from build123d import *

# Parameters (mm, degrees)
SKETCH2_W           = 76
SKETCH2_H           = 178
BOSS_EXTRUDE1_DEPTH = 0.9
SKETCH4_R           = 2.667
CUT_EXTRUDE1_DEPTH  = 2
SKETCH5_R           = 2.667
SKETCH5_R_2         = 1.5
BOSS_EXTRUDE2_DEPTH = 0.254
CHAMFER1_SIZE       = 3


with BuildPart() as part:
    # Sketch2 → Boss-Extrude1 (new body)
    with BuildSketch(Plane.XY):
        with Locations((38, 89)):
            Rectangle(SKETCH2_W, SKETCH2_H)
    extrude(amount=BOSS_EXTRUDE1_DEPTH)

    # Sketch4 → Cut-Extrude1 (cut)
    with BuildSketch(Plane.XY.offset(0.9)):
        with Locations((4, 173)):
            Circle(SKETCH4_R)
        with Locations((72, 173)):
            Circle(SKETCH4_R)
        with Locations((72, 5)):
            Circle(SKETCH4_R)
        with Locations((4, 5)):
            Circle(SKETCH4_R)
    extrude(amount=-CUT_EXTRUDE1_DEPTH, mode=Mode.SUBTRACT)

    # Sketch5 → Boss-Extrude2 (add)
    # profile 1 of 4: a face of its own
    with BuildSketch(Plane.XY.offset(0.9)):
        with Locations((4, 5)):
            Circle(SKETCH5_R)
        with Locations(Location((4, 5, 0), (0, 0, 180))):
            Circle(SKETCH5_R_2, mode=Mode.SUBTRACT)
    # profile 2 of 4: a face of its own
    with BuildSketch(Plane.XY.offset(0.9)):
        with Locations((4, 173)):
            Circle(SKETCH5_R)
        with Locations((4, 173)):
            Circle(SKETCH5_R_2, mode=Mode.SUBTRACT)
    # profile 3 of 4: a face of its own
    with BuildSketch(Plane.XY.offset(0.9)):
        with Locations((72, 5)):
            Circle(SKETCH5_R)
        with Locations((72, 5)):
            Circle(SKETCH5_R_2, mode=Mode.SUBTRACT)
    # profile 4 of 4: a face of its own
    with BuildSketch(Plane.XY.offset(0.9)):
        with Locations((72, 173)):
            Circle(SKETCH5_R)
        with Locations(Location((72, 173, 0), (0, 0, 180))):
            Circle(SKETCH5_R_2, mode=Mode.SUBTRACT)
    extrude(amount=-BOSS_EXTRUDE2_DEPTH)

    # Chamfer1
    chamfer1_edges = [part.edges().sort_by_distance(p)[0] for p in [
        (0, 178, 0.45),
        (76, 178, 0.45),
        (76, 0, 0.45),
        (0, 0, 0.45),
    ]]
    chamfer(chamfer1_edges, length=CHAMFER1_SIZE)


solid = part.part
Verification items for the finished model (mm, model axes). A direction names the side the tool comes from. Round coordinates to 2 decimals unless told otherwise and drop trailing zeros.
1. Release check for a two-part mould opening along Y. For faces 1 (the flat face through (37, 90, 0)), 2 (the cylindrical face through (73.43, 175.25, 0.33)), 3 (the flat face through (1.5, 1.5, 0.4)) record: +Y half, -Y half, draft (parallel to the pull), parting line (faces both ways), or undercut.
Final values:
face 1: draft
face 2: undercut
face 3: -Y half
2. Thickness scan on L1, parallel to X at y = 173, z = 0.35; L2, parallel to Y at x = 72, z = 0.8; L3, parallel to Y at x = 72, z = 0.45. Record the ranges inside material, lowest first.
Final values:
L1: x = 0 to 1.33, 6.67 to 69.33, 74.67 to 76
L2: y = 0 to 3.5, 6.5 to 171.5, 174.5 to 178
L3: y = 0 to 2.33, 7.67 to 170.33, 175.67 to 178
3. Go/stop test with a flat-tipped pin: P1, Ø2.5, axis at x = 4.5, y = 5, coming from the -Z side. Record where the tip stops, or that it passes through.
Final values:
P1: stops at z = 0.65
4. Access from +Z, -Z, +X, -X, +Y, -Y to the whole of each face (thin tool, end or side, straight path). Record for faces 4 (the flat face through (74.5, 1.5, 0.4)), 5 (the flat face through (72, 171, 0.646)).
Final values:
face 4: +Z, -Z, +X, -Y
face 5: -Z
